Design review of the part built by this model. Coordinates are the model's own, in mm. Face numbers are marked on the shaded views. A direction names the side the tool comes from. Give positions to 0.01 mm unless a question says otherwise; leave off trailing zeros. Order: outer loops, then holes, each group sorted by start corner. A loop starts at its lowest first (then second) coordinate and runs counter-clockwise, first axis right, second up. Notation, with made-up numbers: (-20, 80) -> (-11, 80) arc R11 cw to (-11, 89) -> close; hole circle Ø11 at (-10, 19.25). An arc over 180 degrees is marked (long way). One line per item, written item: value. Start each with the question number.
1) Wall thickness on line 1 along Y through (x, z) = (0, -1); line 2 along Y through (x, z) = (-6, 1.9); line 3 along Y through (x, z) = (7.5, 1.4): over which ranges is each line inside the solid? List them lowest first. Write a range as from..to.
2) Consider section A-A (z = 0.55). State the section outline as (x, y) points.
3) The part is to be moulded in two halves that separate along Y. For the marked faces 4 and 5, say which applies: released by +Y, released by -Y, zero draft, split by the parting line, or undercut.
4) Consider section B-B (x = 0). State the section outline as (y, z) points.
5) For pin 1 (12.5 mm diameter, centred on x = -6.5, y = 3, fed in from -Z); pin 2 (2 mm diameter, centred on x = 4.5, z = 0.5, fed in from +Y); pin 3 (1.5 mm diameter, centred on x = -6.5, z = 0.5, fed in from +Y), all flat-tipped, find the tip position at first contact; note any pin that passes through.
6) Consider section D-D (z = -2.35). State the section outline as (x, y) points, plus the area to 3 significant figures.
7) Tool access review of the marked faces 1, 2 and 3: name each direction out of +Z, -Z, +X, -X, +Y, -Y from which nothing blocks a thin tool from reaching the whole face with its end or side.
8) Consider section C-C (y = 0). State the section outline as (x, z) points, plus the area to 4 significant figures.
from build123d import *
from build123d.topology import SkipClean

# Parameters (mm, degrees)
SKETCH1_R           = 10.85
BOSS_EXTRUDE1_DEPTH = 2
SKETCH2_R           = 14
BOSS_EXTRUDE2_DEPTH = 1
BOSS_EXTRUDE3_START = 5
BOSS_EXTRUDE3_DEPTH = 5


with BuildPart() as part:
    # Sketch1 → Boss-Extrude1 (new body)
    with BuildSketch(Plane.XY):
        Circle(SKETCH1_R)
    extrude(amount=BOSS_EXTRUDE1_DEPTH)

    # Sketch2 → Boss-Extrude2 (add)
    with BuildSketch(Plane.XY.offset(2)):
        Circle(SKETCH2_R)
    extrude(amount=BOSS_EXTRUDE2_DEPTH)

    # Sketch3 → Boss-Extrude3 (add)
    with SkipClean():  # the faces are left unmerged after this step: merging them gives an invalid solid
        with BuildSketch(Plane(origin=(0, 0, 2), x_dir=(-1, 0, 0), z_dir=(0, 0, -1)).offset(BOSS_EXTRUDE3_START)):
            with BuildLine():
                ThreePointArc((8.627279255, -9.251624325), (-12.65, 0), (8.627279255, 9.251624325))
                Line((8.627279255, 9.251624325), (9.547977041, 10.238951823))
                ThreePointArc((9.547977041, 10.238951823), (-14, 0), (9.547977041, -10.238951823))
                Line((9.547977041, -10.238951823), (8.627279255, -9.251624325))
            make_face()
        extrude(amount=-BOSS_EXTRUDE3_DEPTH)


solid = part.part
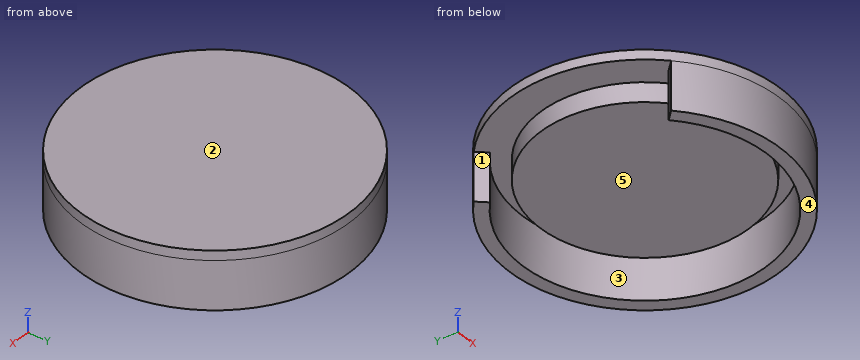
Checked values:
1. line 1: y = -14..-12.65, 12.65..14
1. line 2: y = -12.65..-11.14, -9.04..9.04, 11.14..12.65
1. line 3: y = -11.82..-10.19, -7.84..7.84, 10.19..11.82
2. outline: circle Ø21.7 at (0, 0); (-9.55, -10.24) arc R14 ccw (long way) to (-9.55, 10.24) -> (-8.63, 9.25) arc R12.65 cw (long way) to (-8.63, -9.25) -> close
3. face 4: zero draft
3. face 5: undercut
4. outline: (-14, -3) -> (-12.65, -3) -> (-12.65, 2) -> (-10.85, 2) -> (-10.85, 0) -> (10.85, 0) -> (10.85, 2) -> (12.65, 2) -> (12.65, -3) -> (14, -3) -> (14, 3) -> (-14, 3) -> close
5. pin 1: stops at z = 0
5. pin 2: stops at y = 13.56
5. pin 3: stops at y = 12.76
6. outline: (-9.55, -10.24) arc R14 ccw (long way) to (-9.55, 10.24) -> (-8.63, 9.25) arc R12.65 cw (long way) to (-8.63, -9.25) -> close
6. area: 83.5 mm^2
7. face 1: -Z, -X
7. face 2: +Z, +X, -X, +Y, -Y
7. face 3: -Z
8. outline: (-14, 2) -> (-10.85, 2) -> (-10.85, 0) -> (10.85, 0) -> (10.85, 2) -> (12.65, 2) -> (12.65, -3) -> (14, -3) -> (14, 3) -> (-14, 3) -> close
8. area: 78.15 mm^2
